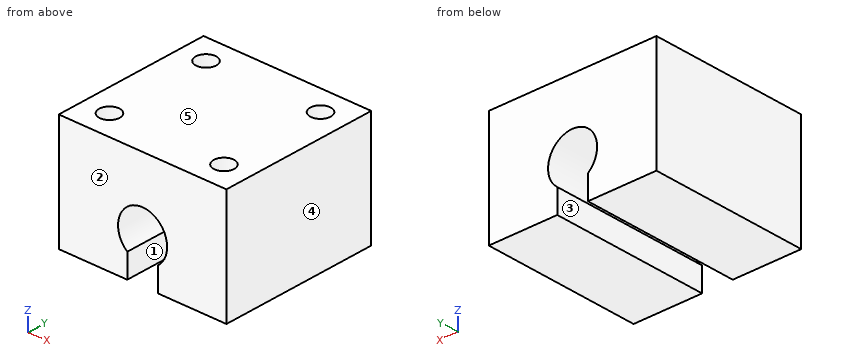
```python
from build123d import *

# Parameters (mm, degrees)
SKETCH_W        = 41
SKETCH_H        = 28
PAD_DEPTH       = 39
POCKET_DEPTH    = 39.001
SKETCH002_R     = 2.5
POCKET001_DEPTH = 10


with BuildPart() as part:
    # Sketch → Pad (new body)
    with BuildSketch(Plane.XZ):
        with Locations((20.5, 14)):
            Rectangle(SKETCH_W, SKETCH_H)
    extrude(amount=-PAD_DEPTH)

    # Sketch001 → Pocket (cut, through all)
    with BuildSketch(Plane.XZ):
        with BuildLine():
            ThreePointArc((24.25, 5.816252), (20.5, 16.5), (16.75, 5.816252))
            Line((16.75, 5.816252), (16.75, 0))
            Line((16.75, 0), (24.25, 0))
            Line((24.25, 5.816252), (24.25, 0))
        make_face()
    extrude(amount=-POCKET_DEPTH, mode=Mode.SUBTRACT)

    # Sketch002 → Pocket001 (cut)
    with BuildSketch(Plane(origin=(0, 0, 28), x_dir=(-1, 0, 0), z_dir=(0, 0, 1))):
        with Locations((-34.5, -6.5)):
            Circle(SKETCH002_R)
        with Locations((-6.5, -6.5)):
            Circle(SKETCH002_R)
        with Locations((-34.5, -32.5)):
            Circle(SKETCH002_R)
        with Locations((-6.5, -32.5)):
            Circle(SKETCH002_R)
    extrude(amount=-POCKET001_DEPTH, mode=Mode.SUBTRACT)


solid = part.part
```
Can you work these out from the model? Positions are in its coordinate system, mm. Face numbers are marked on the shaded views. A direction names the side the tool comes from. Round coordinates to 2 decimals unless told otherwise and drop trailing zeros. Loops run counter-clockwise (first coordinate to the right, second up) from the corner with the lowest first, then second, coordinate; pieces in that order, holes last.
Item 1: Suppose I cut it at C-C, the plane y = 22. Write out the boundary of the cut face in (x, z), then the cut area to 3 significant figures.
Item 2: Suppose I cut it at B-B, the plane z = 10.5. Write out the boundary of the cut face in (x, y), then the cut area to 3 significant figures.
Item 3: If we mould it in two halves opening along X, with no side actions, what happens to the marked faces 3, 4 and 5? For each: +X half, -X half, draft (parallel to the pull), parting line (faces both ways), or undercut.
Item 4: Will these pins go through, and if not, where does the flat tip stop? pin 1 Ø2 at (x, z) = (27, 18.5) entering from -Y; pin 2 Ø9.5 at (x, z) = (20.5, 10.5) entering from -Y (3 decimals); pin 3 Ø1.5 at (x, y) = (7.5, 32.5) entering from +Z.
Item 5: Which directions (+Z, -Z, +X, -X, +Y, -Y) give clear straight access to the entire face, cutting with the end or side of a thin tool? Please do the marked faces 1 and 2.
Item 6: Please list where these lines run through material, in increasing order: L1, parallel to Y at x = 34.5, z = 22.5; L2, parallel to X at y = 32.5, z = 25.5; L3, parallel to X at y = 25, z = 4.5.
Item 7: Suppose I cut it at A-A, the plane z = 23.75. Write out the boundary of the cut face in (x, y).
Item 8: Suppose I cut it at D-D, the plane x = 33.5. Write out the boundary of the cut face in (y, z).
Reported:
1. outline: (0, 0) - (16.75, 0) - (16.75, 5.82) arc R6 cw (long way) to (24.25, 5.82) - (24.25, 0) - (41, 0) - (41, 28) - (0, 28) - close
1. area: 998 mm2
2. outline: (0, 0) - (14.5, 0) - (14.5, 39) - (0, 39) - close; (26.5, 0) - (41, 0) - (41, 39) - (26.5, 39) - close
2. area: 1,130 mm2
3. face 3: undercut
3. face 4: +X half
3. face 5: draft
4. pin 1: stops at y = 0
4. pin 2: passes through
4. pin 3: stops at z = 18
5. face 1: -Z, +Y, -Y
5. face 2: +Z, -Z, +X, -X, -Y
6. L1: y = 0 to 4, 9 to 30, 35 to 39
6. L2: x = 0 to 4, 9 to 32, 37 to 41
6. L3: x = 0 to 16.75, 24.25 to 41
7. outline: (0, 0) - (41, 0) - (41, 39) - (0, 39) - close; hole circle Ø5 at (6.5, 6.5); hole circle Ø5 at (6.5, 32.5); hole circle Ø5 at (34.5, 6.5); hole circle Ø5 at (34.5, 32.5)
8. outline: (0, 0) - (39, 0) - (39, 28) - (34.79, 28) - (34.79, 18) - (30.21, 18) - (30.21, 28) - (8.79, 28) - (8.79, 18) - (4.21, 18) - (4.21, 28) - (0, 28) - close
